For this review, take the finished solid that the model builds, in its own axes (mm). Coordinates: 2 decimals unless noted, no trailing zeros. Order: outer loops, then holes, each group sorted by start corner. A loop starts at its lowest first (then second) coordinate and runs counter-clockwise, first axis right, second up. Notation, with made-up numbers: M 41.25,-9.75 L 62.25,-9.75 A13 cw 62.25,-2.75 Z; hole C -25.75,40 d9. An arc over 180 degrees is marked long. Use one line per item in the form item = value. Start each with the question number.
```python
from build123d import *

# Parameters (mm, degrees)
SKETCH1_R           = 75.9206
BOSS_EXTRUDE1_DEPTH = 12.7
SKETCH1_10_R        = 40.4114
CUT_EXTRUDE2_DEPTH  = 13.7
CUT_EXTRUDE3_DEPTH  = 13.7


with BuildPart() as part:
    # Sketch1 → Boss-Extrude1 (new body)
    with BuildSketch(Plane(origin=(0, 0, 0), x_dir=(1, 0, 0), z_dir=(0, 1, 0))):
        Circle(SKETCH1_R)
    extrude(amount=BOSS_EXTRUDE1_DEPTH)

    # Sketch1<10> → Cut-Extrude2 (cut, through all)
    with BuildSketch(Plane(origin=(0, 0, 0), x_dir=(1, 0, 0), z_dir=(0, 1, 0))):
        Circle(SKETCH1_10_R)
    extrude(amount=CUT_EXTRUDE2_DEPTH, mode=Mode.SUBTRACT)

    # Sketch2 → Cut-Extrude3 (cut, through all)
    with BuildSketch(Plane(origin=(0, 12.7, 0), x_dir=(1, 0, 0), z_dir=(0, 1, 0))):
        with BuildLine():
            Line((76.2, 12.7), (76.2, -12.7))
            ThreePointArc((76.2, -12.7), (63.217526972, 0), (76.2, 12.7))
        make_face()
    extrude(amount=-CUT_EXTRUDE3_DEPTH, mode=Mode.SUBTRACT)


solid = part.part
```
1. Consider section C-C, the plane y = 8.75. Write out the cut boundary in (x, z).
2. Consider section D-D, the plane z = -44. Write out the cut boundary in (x, y), plus the area to 3 significant figures.
3. To check wall thickness, follow line 1 (Z direction, x = 0, y = 5.25); line 2 (Z direction, x = 24, y = 1.75); line 3 (X direction, y = 7.5, z = 17.5). State the ranges of each line that lie inside material, in increasing order.
4. Consider section B-B, the plane x = 0. Write out the cut boundary in (y, z).
5. Consider section A-A, the plane z = 0. Write out the cut boundary in (x, y), plus the area to 3 significant figures.
6. For pin 1 Ø4 at (x, y) = (-3, 6.5) entering from +Z; pin 2 Ø1.5 at (x, y) = (-17, 2) entering from -Z; pin 3 Ø3 at (x, y) = (-57.5, 6.5) entering from +Z, all flat-tipped, find the tip position at first contact; note any pin that passes through.
Answers follow:
q1.outline = M 74.86,-12.66 A12.7 cw 74.86,12.66 A75.92 ccw long Z; hole C 0,0 d80.82
q2.outline = M -61.87,0 L 61.87,0 L 61.87,12.7 L -61.87,12.7 Z
q2.area = 1,570 mm²
q3.line_1 = -75.92 to -40.41, 40.41 to 75.92
q3.line_2 = -72.03 to -32.51, 32.51 to 72.03
q3.line_3 = -73.88 to -36.43, 36.43 to 73.88
q4.outline = M 0,-75.92 L 12.7,-75.92 L 12.7,-40.41 L 0,-40.41 Z; M 0,40.41 L 12.7,40.41 L 12.7,75.92 L 0,75.92 Z
q5.outline = M -75.92,0 L -40.41,0 L -40.41,12.7 L -75.92,12.7 Z; M 40.41,0 L 63.22,0 L 63.22,12.7 L 40.41,12.7 Z
q5.area = 741 mm²
q6.pin_1 = 75.91
q6.pin_2 = -74.16
q6.pin_3 = 51.26
